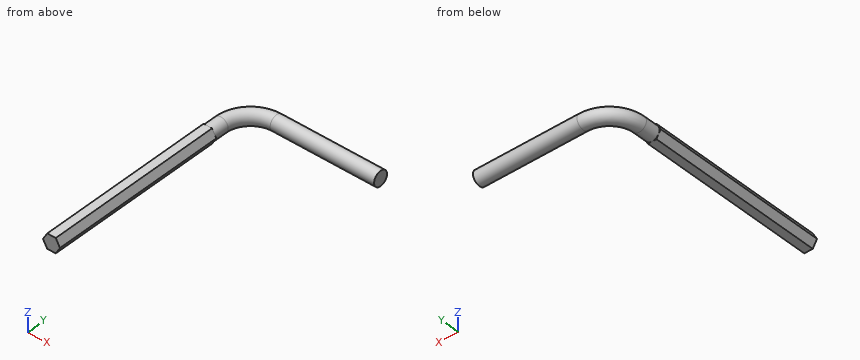
from build123d import *

# Parameters (mm, degrees)
SKETCH16_R          = 2.475
BOSS_EXTRUDE2_DEPTH = 60


with BuildPart() as part:
    # Sweep4: sweep along a path in Sketch15
    with BuildLine(Plane.XY) as sweep4_path:
        Line((0, 0), (0, 65))
        ThreePointArc((0, 65), (2.928932188, 72.071067812), (10, 75))
        Line((10, 75), (45, 75))
    # Sketch16 → Sweep4 (sweep)
    with BuildSketch(Plane(origin=(0, 0, 0), x_dir=(1, 0, 0), z_dir=(0, 1, 0))):
        Circle(SKETCH16_R)
    sweep(path=sweep4_path.line)

    # Sketch18 → Boss-Extrude2 (add)
    with BuildSketch(Plane(origin=(0, 0, 0), x_dir=(1, 0, 0), z_dir=(0, 1, 0))):
        Polygon((2.857883832, 0), (1.428941916, 2.475), (-1.428941916, 2.475), (-2.857883832, 0), (-1.428941916, -2.475), (1.428941916, -2.475), align=None)
    extrude(amount=BOSS_EXTRUDE2_DEPTH)


solid = part.part
For this review, take the finished solid that the model builds, in its own axes (mm). Round coordinates to 2 decimals unless told otherwise and drop trailing zeros. Write each loop counter-clockwise with the first axis right and the second up, starting at its lowest first coordinate (ties: lowest second). Pieces come first, ordered by that corner, then holes. Notation, with made-up numbers: (-30.75, 21.25) - (-22.75, 21.25) arc R22 cw to (-22.75, 36.25) - close; hole circle Ø4 at (33, -39.75). An arc over 180 degrees is marked (long way). Write item = value, one per line. Start each with the question number.
1. For pin 1 Ø0.6 at (x, z) = (1, -1.5) entering from +Y; pin 2 Ø1 at (x, y) = (4, 29) entering from -Z; pin 3 Ø0.8 at (x, z) = (2.5, -0.5) entering from +Y; pin 4 Ø1 at (x, z) = (1, 2) entering from +Y, all flat-tipped, find the tip position at first contact; note any pin that passes through.
2. Wall thickness on L1, parallel to Y at x = 32, z = -0.3; L2, parallel to X at y = 61, z = 0.25; L3, parallel to X at y = 22, z = 1.25: over which ranges is each line inside the solid? List them lowest first.
3. Consider section A-A on y = 9. State the section outline as (x, z) points (3 decimals).
4. Consider section B-B on x = 32. State the section outline as (y, z) points (3 decimals), plus the area to 3 significant figures.
Evaluation:
q1.pin_1 = 73.34
q1.pin_2 = through
q1.pin_3 = 75.21
q1.pin_4 = 73.1
q2.L1 = 72.54 to 77.46
q2.L2 = -2.46 to 2.46
q2.L3 = -2.14 to 2.14
q3.outline = (-2.858, 0) - (-1.429, -2.475) - (1.429, -2.475) - (2.858, 0) - (1.429, 2.475) - (-1.429, 2.475) - close
q4.outline = circle Ø4.95 at (75, 0)
q4.area = 19.2 mm2
